Autodesk Inventor part; units mm, degrees
ref_plane "YZ Plane" through (0, 0, 0) normal (1, 0, 0) x (0, 1, 0)
ref_plane "XZ Plane" through (0, 0, 0) normal (0, 1, 0) x (-1, 0, 0)
ref_plane "XY Plane" through (0, 0, 0) normal (0, 0, 1) x (1, 0, 0)
sketch "Sketch1" plane through (0, 0, 0) normal (0, 0, 1) x (1, 0, 0)
  circle A0 centre (0, 0) radius 22.5
  line L0 (162.5, 0) -> (-22.5, 0) construction
  circle A1 centre (0, 0) radius 5
  line L1 (60, 10) -> (20.1556, 10)
  line L2 (20.1556, 10) -> (20.1556, -10)
  line L3 (20.1556, -10) -> (60, -10)
  line L4 (60, -10) -> (60, 10)
  circle A2 centre (47, 0) radius 3
  point P0 (6.3, 21.6)
  point P1 (60, 0)
  dimension "d0" = 45
  dimension "d3" = 10
  dimension "d7" = 20
  dimension "d8" = 60
  dimension "d9" = 6
  dimension "d10" = 13
extrude "Extrusion1" add sketch "Sketch1" along normal mid plane 2
fillet "Fillet1" radius 5 2 edges at (20.1556, 10, 0) (20.1556, -10, 0)
fillet "Fillet2" radius 2 2 edges at (60, -10, 0) (60, 10, 0)
properties part number "stelscharnier onderkant" material "Stainless Steel"
Input: part model. Units: mm. Frame: model coordinates. A direction names the side the tool comes from. Coordinates: 2 decimals unless noted, no trailing zeros. Write each loop counter-clockwise with the first axis right and the second up, starting at its lowest first coordinate (ties: lowest second). Pieces come first, ordered by that corner, then holes. Notation, with made-up numbers: (24, 55.5) -> (29, 55.5) arc R22 cw to (29, 85.5) -> close; hole circle Ø1 at (34, 45.25). An arc over 180 degrees is marked (long way). Answer as a JSON object with one key per item and string values.
1. Material intervals for line 1 (Y direction, x = 47, z = -0.2); line 2 (Y direction, x = 0, z = 0.2); line 3 (Y direction, x = 34, z = -0.9), sorted ascending. Write a range as from..to.
Result set:
{"line 1": "y = -10..-3, 3..10", "line 2": "y = -22.5..-5, 5..22.5", "line 3": "y = -10..10"}
2. Section D-D on x = 47. Return the cut outline in (y, z), then the cut area to 3 significant figures.
Result set:
{"outline": "(-10, -1) -> (-3, -1) -> (-3, 1) -> (-10, 1) -> close; (3, -1) -> (10, -1) -> (10, 1) -> (3, 1) -> close", "area": "28.0 mm2"}
3. Section C-C on z = 0.4. Return the cut outline in (x, y), then the cut area to 3 significant figures.
Result set:
{"outline": "(18.86, -12.27) arc R5 cw to (23.05, -10) -> (58, -10) arc R2 ccw to (60, -8) -> (60, 8) arc R2 ccw to (58, 10) -> (23.05, 10) arc R5 cw to (18.86, 12.27) arc R22.5 ccw (long way) to start; hole circle Ø10 at (0, 0); hole circle Ø6 at (47, 0)", "area": "2,250 mm2"}
4. Section A-A on x = 0. Return the cut outline in (y, z), then the cut area to 3 significant figures.
Result set:
{"outline": "(-22.5, -1) -> (-5, -1) -> (-5, 1) -> (-22.5, 1) -> close; (5, -1) -> (22.5, -1) -> (22.5, 1) -> (5, 1) -> close", "area": "70.0 mm2"}
5. Mould query, pull axis Y, two halves, no side actions, for faces 4 (the face through (44, 0, 0)), 5 (the face through (20.635, 10.621, 0.014)), 6 (the face through (9, 0, 1)), 7 (the face through (-1.08, 4.88, -0.01)). Classes: released by +Y, released by -Y, zero draft, split by the parting line, or undercut.
Result set:
{"face 4": "undercut", "face 5": "released by +Y", "face 6": "zero draft", "face 7": "undercut"}
6. First-contact query: P1, Ø1, axis at x = 48, y = -0.5, coming from the -Z side. Flat tip, straight axial feed; report the tip coordinate or a pass-through.
Result set:
{"P1": "passes through"}
7. Access query for faces 1 (the face through (40, -10, 0)), 2 (the face through (9, 0, -1)), 3 (the face through (41, 10, 0)). Directions: +Z, -Z, +X, -X, +Y, -Y. A direction counts if a zero-diameter tool reaches every point of the face in a straight line with its end or side. Return the directions, or none.
Result set:
{"face 1": "+Z, -Z, +X, -Y", "face 2": "-Z, +X, -X, +Y, -Y", "face 3": "+Z, -Z, +X, +Y"}
8. Section B-B on y = 0. Return the cut outline in (x, z).
Result set:
{"outline": "(-22.5, -1) -> (-5, -1) -> (-5, 1) -> (-22.5, 1) -> close; (5, -1) -> (44, -1) -> (44, 1) -> (5, 1) -> close; (50, -1) -> (60, -1) -> (60, 1) -> (50, 1) -> close"}
